```python
from build123d import *

# Parameters (mm, degrees)
EXTRUDE_1_DEPTH             = 15
SKETCH_2_W                  = 1
SKETCH_2_H                  = 1
CUT_EXTRUDE_1_DEPTH         = 15
SKETCH_6_W                  = 5
SKETCH_6_H                  = 1.75
EXTRUDE_2_DEPTH             = 7.5
SKETCH_7_W                  = 5
SKETCH_7_H                  = 1.75
EXTRUDE_3_DEPTH             = 7.5
HOLE_WIZARD_M21_D           = 2.2
HOLE_WIZARD_M21_CSINK_D     = 4.4
HOLE_WIZARD_M21_CSINK_ANGLE = 90
CUT_EXTRUDE_2_DEPTH         = 1.2
SKETCH_8_W                  = 2.7
SKETCH_8_H                  = 1.5
EXTRUDE_4_DEPTH             = 5


with BuildPart() as part:
    # Эскиз1 → Бобышка-Вытянуть1 (new body)
    with BuildSketch(Plane(origin=(0, 0, 0), x_dir=(0, 0, -1), z_dir=(1, 0, 0))):
        with BuildLine():
            Line((0, 2.5), (0, -2.5))
            Line((0, -2.5), (7.8, -2.5))
            ThreePointArc((7.8, -2.5), (5.3, 0), (7.8, 2.5))
            Line((7.8, 2.5), (0, 2.5))
        make_face()
    extrude(amount=EXTRUDE_1_DEPTH)

    # Эскиз2 → Вырез-Вытянуть1 (cut)
    with BuildSketch(Plane(origin=(15, 0, 0), x_dir=(0, 0, -1), z_dir=(1, 0, 0))):
        with Locations((7.3, 2)):
            Rectangle(SKETCH_2_W, SKETCH_2_H)
        with Locations((7.3, -2)):
            Rectangle(SKETCH_2_W, SKETCH_2_H)
    extrude(amount=-CUT_EXTRUDE_1_DEPTH, mode=Mode.SUBTRACT)

    # Эскиз6 → Бобышка-Вытянуть2 (add)
    with BuildSketch(Plane.ZY):
        with Locations((-2.5, 1.625)):
            Rectangle(SKETCH_6_W, SKETCH_6_H)
        with Locations((-2.5, -1.625)):
            Rectangle(SKETCH_6_W, SKETCH_6_H)
    extrude(amount=EXTRUDE_2_DEPTH)

    # Эскиз7 → Бобышка-Вытянуть3 (add)
    with BuildSketch(Plane(origin=(15, 0, 0), x_dir=(0, 0, -1), z_dir=(1, 0, 0))):
        with Locations((2.5, 1.625)):
            Rectangle(SKETCH_7_W, SKETCH_7_H)
        with Locations((2.5, -1.625)):
            Rectangle(SKETCH_7_W, SKETCH_7_H)
    extrude(amount=EXTRUDE_3_DEPTH)

    # Зенковка для винта с полупотайной головкой M21 (through all)
    with Locations(Plane(origin=(0, 2.5, 0), x_dir=(1, 0, 0), z_dir=(0, 1, 0))):
        with Locations((20, 2.5), (-5, 2.5)):
            CounterSinkHole(HOLE_WIZARD_M21_D / 2, HOLE_WIZARD_M21_CSINK_D / 2, counter_sink_angle=HOLE_WIZARD_M21_CSINK_ANGLE)

    # Эскиз5 → Вырез-Вытянуть2 (cut)
    with BuildSketch(Plane.XZ.offset(2.5)):
        Polygon((-6.178867871, -0.458141777), (-7.357735027, -2.500000412), (-6.178867157, -4.541858635), (-3.821132129, -4.541858223), (-2.642264973, -2.499999588), (-3.821132843, -0.458141365), align=None)
        Polygon((21.178867119, -4.541858635), (18.821132092, -4.541858223), (17.642264935, -2.499999588), (18.821132806, -0.458141365), (21.178867833, -0.458141777), (22.357734989, -2.500000412), align=None)
    extrude(amount=-CUT_EXTRUDE_2_DEPTH, mode=Mode.SUBTRACT)

    # Эскиз8 → Бобышка-Вытянуть4 (add)
    with BuildSketch(Plane.XY):
        with Locations((-1.35, 0)):
            Rectangle(SKETCH_8_W, SKETCH_8_H)
        with Locations((16.35, 0)):
            Rectangle(SKETCH_8_W, SKETCH_8_H)
    extrude(amount=-EXTRUDE_4_DEPTH)


solid = part.part
```
Source: CAD feature listing. Evaluate the final solid. Frame: model axes, mm. A direction names the side the tool comes from. Round coordinates to 2 decimals unless told otherwise and drop trailing zeros. Write each loop counter-clockwise with the first axis right and the second up, starting at its lowest first coordinate (ties: lowest second). Pieces come first, ordered by that corner, then holes. Notation, with made-up numbers: M 9.25,19 L 14.25,19 A21 cw 14.25,34 Z; hole C 54.25,7.5 d3. An arc over 180 degrees is marked long. Use CSV: the item, a comma, the result in double quotes. Start each with the question number.
Q1. Pull-direction query (Z, two-part tool) for faces 4 (the face through (19, 1, -5)), 5 (the face through (7, -2.5, -3)), 6 (the face through (-3.9, -1, -2.5)); classes: +Z half, -Z half, draft (parallel to the pull), parting line (faces both ways), or undercut.
Q2. Cut plane B-B on y = 1.95. Output: boundary loops of the cut face in (x, z), plus the area to 3 significant figures.
Q3. Cut plane D-D on x = 11.5. Output: boundary loops of the cut face in (y, z), plus the area to 3 significant figures.
Q4. Cut plane C-C on z = -5.75. Output: boundary loops of the cut face in (x, y), plus the area to 3 significant figures.
Q5. Cut plane A-A on x = 20. Output: boundary loops of the cut face in (y, z), plus the area to 3 significant figures.
Q6. Access query for faces 1 (the face through (21.1, 1.1, -2.5)), 2 (the face through (20, 0.75, -1)), 3 (the face through (20, -2, -4.542)). Directions: +Z, -Z, +X, -X, +Y, -Y. A direction counts if a zero-diameter tool reaches every point of the face in a straight line with its end or side. Return the directions, or none.
Q7. First-contact query: P1, Ø2, axis at x = 20, z = -2.5, coming from the -Y side; P2, Ø1.2, axis at y = 0, z = -2.5, coming from the -X side; P3, Ø3, axis at x = 20, z = -2.5, coming from the +Y side; P4, Ø0.8, axis at y = 0, z = -3.5, coming from the +X side. Flat tips, straight axial feed; report the tip coordinate or a pass-through.
Q8. Line query: line 1 (Z direction, x = 20, y = 0.95); line 2 (Z direction, x = 19.5, y = -2.15); line 3 (X direction, y = -2, z = -4). Output: solid intervals per line, ascending. Write a range as from..to.
Results found:
1,face 4,"-Z half"
1,face 5,"draft"
1,face 6,"undercut"
2,outline,"M -7.5,-5 L 0,-5 L 0,-6.24 L 15,-6.24 L 15,-5 L 22.5,-5 L 22.5,0 L -7.5,0 Z; hole C -5,-2.5 d3.3; hole C 20,-2.5 d3.3"
2,area,"151 mm^2"
3,outline,"M -2.5,-6.8 L -2.29,-6.8 A2.5 cw 2.29,-6.8 L 2.5,-6.8 L 2.5,0 L -2.5,0 Z"
3,area,"29.0 mm^2"
4,outline,"M 0,-2.5 L 15,-2.5 L 15,-1.43 L 0,-1.43 Z; M 0,1.43 L 15,1.43 L 15,2.5 L 0,2.5 Z"
4,area,"32.1 mm^2"
5,outline,"M -2.5,-5 L -0.75,-5 L -0.75,-3.6 L -1.3,-3.6 L -1.3,-4.54 L -2.5,-4.54 Z; M -2.5,-0.46 L -1.3,-0.46 L -1.3,-1.4 L -0.75,-1.4 L -0.75,0 L -2.5,0 Z; M 0.75,-5 L 2.5,-5 L 2.5,-4.7 L 1.4,-3.6 L 0.75,-3.6 Z; M 0.75,-1.4 L 1.4,-1.4 L 2.5,-0.3 L 2.5,0 L 0.75,0 Z"
5,area,"6.33 mm^2"
6,face 1,"+Y, -Y"
6,face 2,"+Z, -Z, +X"
6,face 3,"-Y"
7,P1,"through"
7,P2,"x = -2.7"
7,P3,"y = 1.8"
7,P4,"x = 17.7"
8,line 1,"-5..-3.6, -1.4..0"
8,line 2,"-5..-4.54, -0.46..0"
8,line 3,"-7.5..-6.49, -3.51..18.51, 21.49..22.5"
